from build123d import *

# Parameters (mm, degrees)
SKETCH1_W           = 34
SKETCH1_H           = 35.6
BOSS_EXTRUDE1_DEPTH = 2.2
BOSS_EXTRUDE2_DEPTH = 3
BOSS_EXTRUDE3_START = -32
BOSS_EXTRUDE3_DEPTH = 2
SKETCH4_R           = 2.5
SKETCH4_R_2         = 1.5
CUT_EXTRUDE1_DEPTH  = 12
SKETCH4_3_R         = 10.925
SKETCH4_3_R_2       = 1.5
SKETCH4_3_R_3       = 2.5
CUT_EXTRUDE2_DEPTH  = 2.2
SKETCH5_R           = 4
CUT_EXTRUDE3_DEPTH  = 12.2


with BuildPart() as part:
    # Sketch1 → Boss-Extrude1 (new body)
    with BuildSketch(Plane(origin=(0, 0, 0), x_dir=(1, 0, 0), z_dir=(0, 1, 0))):
        Rectangle(SKETCH1_W, SKETCH1_H)
    extrude(amount=BOSS_EXTRUDE1_DEPTH)

    # Sketch3 → Boss-Extrude2 (add)
    with BuildSketch(Plane.ZY.offset(17)):
        with BuildLine():
            Line((0, 37.8), (0, 2.2))
            Line((0, 2.2), (17.8, 2.2))
            Line((17.8, 2.2), (17.8, 20))
            ThreePointArc((17.8, 20), (12.586500705, 32.586500705), (0, 37.8))
        make_face()
        with BuildLine():
            Line((-17.8, 2.2), (0, 2.2))
            Line((0, 2.2), (0, 37.8))
            ThreePointArc((0, 37.8), (-12.586500705, 32.586500705), (-17.8, 20))
            Line((-17.8, 20), (-17.8, 2.2))
        make_face()
    extrude(amount=-BOSS_EXTRUDE2_DEPTH)

    # Sketch3<4> → Boss-Extrude3 (add)
    with BuildSketch(Plane.ZY.offset(17).offset(BOSS_EXTRUDE3_START)):
        with BuildLine():
            Line((-17.8, 2.2), (0, 2.2))
            Line((0, 2.2), (0, 37.8))
            ThreePointArc((0, 37.8), (-12.586500705, 32.586500705), (-17.8, 20))
            Line((-17.8, 20), (-17.8, 2.2))
        make_face()
        with BuildLine():
            Line((0, 37.8), (0, 2.2))
            Line((0, 2.2), (17.8, 2.2))
            Line((17.8, 2.2), (17.8, 20))
            ThreePointArc((17.8, 20), (12.586500705, 32.586500705), (0, 37.8))
        make_face()
    extrude(amount=-BOSS_EXTRUDE3_DEPTH)

    # Sketch4 → Cut-Extrude1 (cut)
    with BuildSketch(Plane.ZY.offset(17)):
        with Locations((0, 20)):
            Circle(SKETCH4_R)
        with Locations((7, 20)):
            Circle(SKETCH4_R_2)
        with Locations((0, 27)):
            Circle(SKETCH4_R_2)
        with Locations((-7, 20)):
            Circle(SKETCH4_R_2)
        with Locations((0, 13)):
            Circle(SKETCH4_R_2)
    extrude(amount=-CUT_EXTRUDE1_DEPTH, mode=Mode.SUBTRACT)

    # Sketch4<3> → Cut-Extrude2 (cut)
    with BuildSketch(Plane.ZY.offset(17)):
        with Locations((0, 20)):
            Circle(SKETCH4_3_R)
        with Locations((0, 27)):
            Circle(SKETCH4_3_R_2, mode=Mode.SUBTRACT)
        with Locations((0, 13)):
            Circle(SKETCH4_3_R_2, mode=Mode.SUBTRACT)
        with Locations((-7, 20)):
            Circle(SKETCH4_3_R_2, mode=Mode.SUBTRACT)
        with Locations((7, 20)):
            Circle(SKETCH4_3_R_2, mode=Mode.SUBTRACT)
        with Locations((0, 20)):
            Circle(SKETCH4_3_R_3, mode=Mode.SUBTRACT)
    extrude(amount=-CUT_EXTRUDE2_DEPTH, mode=Mode.SUBTRACT)

    # Sketch5 → Cut-Extrude3 (cut)
    with BuildSketch(Plane(origin=(17, 0, 0), x_dir=(0, 0, -1), z_dir=(1, 0, 0))):
        with Locations((0, 20)):
            Circle(SKETCH5_R)
    extrude(amount=-CUT_EXTRUDE3_DEPTH, mode=Mode.SUBTRACT)


solid = part.part
Build history of the part. All positions in model axes, mm. A direction names the side the tool comes from. Give positions to 0.01 mm unless a question says otherwise; leave off trailing zeros. Write each loop counter-clockwise with the first axis right and the second up, starting at its lowest first coordinate (ties: lowest second). Pieces come first, ordered by that corner, then holes. Notation, with made-up numbers: (59, 80.5) - (99, 80.5) arc R5 cw to (99, 85.5) - close; hole circle Ø10 at (41, -24). An arc over 180 degrees is marked (long way). Use one line per item in the form item = value. Start each with the question number.
1. Band-saw the part on B-B on z = 2. Write the cut outline in (x, y).
2. Probe line 1 (Y direction, x = -14.45, z = 0); line 2 (X direction, y = 9, z = -1); line 3 (Y direction, x = 15.55, z = 0). List the from-to ranges inside material, lowest first. Write a range as [from, to].
3. Band-saw the part on C-C on z = -3.5. Write the cut outline in (x, y).
4. 3-axis set-ups, long thin cutter, end or side, ignore diameter. For faces 1 (the face through (-14, 16, 0)), 2 (the face through (16.014, 23.966, 0.521)), 3 (the face through (-15.915, 30.832, -1.422)), 4 (the face through (-14.41, 22.48, -0.33)): which of +Z, -Z, +X, -X, +Y, -Y reach the whole face in a straight line?
5. Drop flat-ended pins along their axis: pin 1 Ø13 at (y, z) = (20, 0) entering from -X; pin 2 Ø1 at (x, y) = (4, 4.5) entering from +Z; pin 3 Ø12 at (x, z) = (-8.5, -7) entering from +Y; pin 4 Ø2.5 at (y, z) = (20, 7) entering from -X. Give the stop position or say it passes through.
6. Band-saw the part on A-A on y = 35.5. Write the cut outline in (x, z), plus the area to 3 significant figures.
7. Two-plate mould, pull along X, no slides. Class faces 5 (the face through (15, 16, 4)), 6 (the face through (-14.41, 21.01, 5.89)), 7 (the face through (-14.8, 20, -3)): released by +X, released by -X, zero draft, split by the parting line, or undercut.
8. Band-saw the part on D-D on y = 27. Write the cut outline in (x, z), plus the area to 3 significant figures.
Conclusion:
q1.outline = (-17, 0) - (17, 0) - (17, 16.54) - (15, 16.54) - (15, 2.2) - (-14, 2.2) - (-14, 18.5) - (-14.8, 18.5) - (-14.8, 9.26) - (-17, 9.26) - close; (-17, 30.74) - (-14.8, 30.74) - (-14.8, 21.5) - (-14, 21.5) - (-14, 37.69) - (-17, 37.69) - close; (15, 23.46) - (17, 23.46) - (17, 37.69) - (15, 37.69) - close
q2.line_1 = [0, 11.5], [14.5, 17.5], [22.5, 25.5], [28.5, 37.8]
q2.line_2 = [-17, -14], [15, 17]
q2.line_3 = [0, 16], [24, 37.8]
q3.outline = (-17, 0) - (17, 0) - (17, 18.06) - (15, 18.06) - (15, 2.2) - (-14, 2.2) - (-14, 37.45) - (-17, 37.45) - (-17, 30.35) - (-14.8, 30.35) - (-14.8, 9.65) - (-17, 9.65) - close; (15, 21.94) - (17, 21.94) - (17, 37.45) - (15, 37.45) - close
q4.face_1 = +Z, -Z, +Y
q4.face_2 = +X
q4.face_3 = -X
q4.face_4 = +X, -X
q5.pin_1 = -14.8
q5.pin_2 = through
q5.pin_3 = 37.19
q5.pin_4 = 15
q6.outline = (-17, -8.75) - (-14, -8.75) - (-14, 8.75) - (-17, 8.75) - close; (15, -8.75) - (17, -8.75) - (17, 8.75) - (15, 8.75) - close
q6.area = 87.5 mm²
q7.face_5 = undercut
q7.face_6 = zero draft
q7.face_7 = released by -X
q8.outline = (-17, -16.37) - (-14, -16.37) - (-14, -1.5) - (-14.8, -1.5) - (-14.8, -8.39) - (-17, -8.39) - close; (-17, 8.39) - (-14.8, 8.39) - (-14.8, 1.5) - (-14, 1.5) - (-14, 16.37) - (-17, 16.37) - close; (15, -16.37) - (17, -16.37) - (17, 16.37) - (15, 16.37) - close
q8.area = 124 mm²
